```python
from build123d import *

# Parameters (mm, degrees)
SKETCH1_R                = 16
SKETCH1_R_2              = 12.5
BOSS_EXTRUDE1_DEPTH      = 4
BOSS_EXTRUDE2_DEPTH      = 0.2
BOSS_EXTRUDE2_DEPTH_BACK = 4.2
SKETCH2_R                = 16
SKETCH2_R_2              = 15.5
SKETCH2_R_3              = 13
SKETCH2_R_4              = 12.5


with BuildPart() as part:
    # Sketch1 → Boss-Extrude1 (new body)
    with BuildSketch(Plane(origin=(0, 0, 0), x_dir=(1, 0, 0), z_dir=(0, 1, 0))):
        with Locations(Location((0, 0, 0), (0, 0, 270))):
            Circle(SKETCH1_R)
        with Locations(Location((0, 0, 0), (0, 0, 270))):
            Circle(SKETCH1_R_2, mode=Mode.SUBTRACT)
    extrude(amount=BOSS_EXTRUDE1_DEPTH)

    # Sketch2 → Boss-Extrude2 (add, two sides: drawn at the far end of the back side and taken through both)
    # profile 1 of 2: a face of its own
    with BuildSketch(Plane(origin=(0, 4, 0), x_dir=(1, 0, 0), z_dir=(0, 1, 0)).offset(-BOSS_EXTRUDE2_DEPTH_BACK)):
        with Locations(Location((0, 0, 0), (0, 0, 270))):
            Circle(SKETCH2_R)
        with Locations(Location((0, 0, 0), (0, 0, 270))):
            Circle(SKETCH2_R_2, mode=Mode.SUBTRACT)
    # profile 2 of 2: a face of its own
    with BuildSketch(Plane(origin=(0, 4, 0), x_dir=(1, 0, 0), z_dir=(0, 1, 0)).offset(-BOSS_EXTRUDE2_DEPTH_BACK)):
        with Locations(Location((0, 0, 0), (0, 0, 270))):
            Circle(SKETCH2_R_3)
        with Locations(Location((0, 0, 0), (0, 0, 270))):
            Circle(SKETCH2_R_4, mode=Mode.SUBTRACT)
    extrude(amount=BOSS_EXTRUDE2_DEPTH + BOSS_EXTRUDE2_DEPTH_BACK)


solid = part.part
```
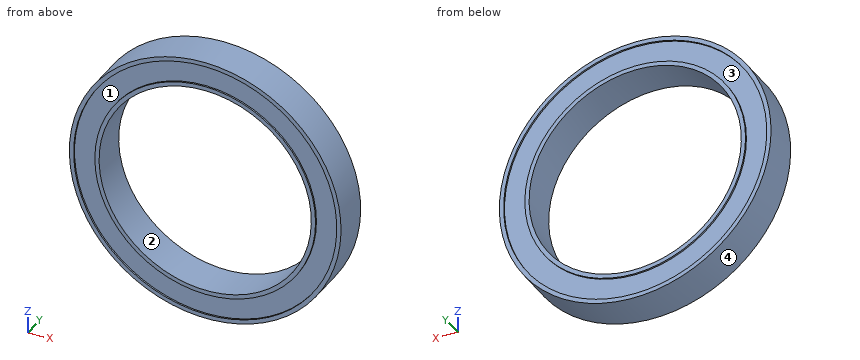
Work out the finished part from the listing and answer in its coordinate system (mm). Face numbers are marked on the shaded views. A direction names the side the tool comes from. Give positions to 0.01 mm unless a question says otherwise; leave off trailing zeros. Order: outer loops, then holes, each group sorted by start corner. A loop starts at its lowest first (then second) coordinate and runs counter-clockwise, first axis right, second up. Notation, with made-up numbers: (27.5, -35) -> (42.5, -35) arc R28 cw to (42.5, -17) -> close; hole circle Ø3 at (80.25, 42). An arc over 180 degrees is marked (long way). Answer as CSV lines item,"result". Start each with the question number.
(1) Section A-A, the plane x = 0 is taken. Write down the section's boundary in (y, z).
(2) Section C-C, the plane y = 1 is taken. Write down the section's boundary in (x, z).
(3) Which of the six approach directions +Z, -Z, +X, -X, +Y, -Y give full straight-line access (tool end or side, diameter ignored) to the marked faces 1 and 2?
(4) Section B-B, the plane z = -12 is taken. Write down the section's boundary in (x, y).
(5) For a pull along X with two mould halves and no side action, classify the marked faces 3 and 4 as released by +X, released by -X, zero draft, split by the parting line, or undercut.
(6) Each of these flat-tipped pins is pushed along its axis until it touches: pin 1 Ø1 at (y, z) = (1, 0.5) entering from -X; pin 2 Ø1.5 at (y, z) = (1, -5.5) entering from -X. Where does it stop, or does it pass through?
(7) Consider line 1 along X through (y, z) = (4.1, 0); line 2 along X through (y, z) = (0.55, -4.5); line 3 along X through (y, z) = (0.2, -4). Determine where each line is inside the solid, lowest interval first.
Entries:
1,outline,"(-0.2, -16) -> (4.2, -16) -> (4.2, -15.5) -> (4, -15.5) -> (4, -13) -> (4.2, -13) -> (4.2, -12.5) -> (-0.2, -12.5) -> (-0.2, -13) -> (0, -13) -> (0, -15.5) -> (-0.2, -15.5) -> close; (-0.2, 12.5) -> (4.2, 12.5) -> (4.2, 13) -> (4, 13) -> (4, 15.5) -> (4.2, 15.5) -> (4.2, 16) -> (-0.2, 16) -> (-0.2, 15.5) -> (0, 15.5) -> (0, 13) -> (-0.2, 13) -> close"
2,outline,"circle Ø32 at (0, 0); hole circle Ø25 at (0, 0)"
3,face 1,"-Y"
3,face 2,"+Y, -Y"
4,outline,"(-10.58, -0.2) -> (-9.81, -0.2) -> (-9.81, 0) -> (-5, 0) -> (-5, -0.2) -> (-3.5, -0.2) -> (-3.5, 4.2) -> (-5, 4.2) -> (-5, 4) -> (-9.81, 4) -> (-9.81, 4.2) -> (-10.58, 4.2) -> close; (3.5, -0.2) -> (5, -0.2) -> (5, 0) -> (9.81, 0) -> (9.81, -0.2) -> (10.58, -0.2) -> (10.58, 4.2) -> (9.81, 4.2) -> (9.81, 4) -> (5, 4) -> (5, 4.2) -> (3.5, 4.2) -> close"
5,face 3,"undercut"
5,face 4,"split by the parting line"
6,pin 1,"x = -16"
6,pin 2,"x = -15.28"
7,line 1,"-16 to -15.5, -13 to -12.5, 12.5 to 13, 15.5 to 16"
7,line 2,"-15.35 to -11.66, 11.66 to 15.35"
7,line 3,"-15.49 to -11.84, 11.84 to 15.49"
